```python
from build123d import *

# Parameters (mm, degrees)
CROQUIS1_W                       = 580
CROQUIS1_H                       = 8.5
CROQUIS4_R                       = 9.75
SALIENTE_EXTRUIR1_DEPTH          = 4
MATRIZL1_COUNT                   = 2
MATRIZL1_PITCH                   = 442
SALIENTE_EXTRUIR3_DEPTH          = 3.8
MATRIZL2_COUNT                   = 2
MATRIZL2_PITCH                   = 40
MATRIZL3_COUNT                   = 2
MATRIZL3_PITCH                   = 332
MATRIZL3_COPY_1_DEPTH            = 3.8
CROQUIS6_R                       = 8.5
SALIENTE_EXTRUIR4_DEPTH          = 3.8
MATRIZL4_COUNT                   = 2
MATRIZL4_PITCH                   = 40
MATRIZL5_COUNT                   = 2
MATRIZL5_PITCH                   = 110
MATRIZL5_COPY_1_SKETCH_R         = 8.5
MATRIZL5_COPY_1_DEPTH            = 3.8
CROQUIS7_R                       = 9.75
CORTAR_EXTRUIR1_DEPTH            = 12
CROQUIS8_R                       = 9.75
SALIENTE_EXTRUIR5_DEPTH          = 4
CROQUIS9_R                       = 8.5
SALIENTE_EXTRUIR6_DEPTH          = 8
CHAFL_N1_SIZE                    = 1
SALIENTE_EXTRUIR7_DEPTH          = 5
SALIENTE_EXTRUIR7_DEPTH_BACK     = 5
CROQUIS10_R                      = 15
CROQUIS11_W                      = 6
CROQUIS11_H                      = 3.35
SALIENTE_EXTRUIR8_DEPTH          = 40
CORTAR_EXTRUIR2_START            = -68.25
CROQUIS12_R                      = 42.065931182
CORTAR_EXTRUIR2_DEPTH            = 68.25
TALADRO_DE_MARGEN_PARA_M71_D     = 7.6
TALADRO_DE_MARGEN_PARA_M71_DEPTH = 30
TALADRO_DE_MARGEN_PARA_M71_TIP   = 2.283270352


with BuildPart() as part:
    # Croquis1 → Revolución1 (revolve)
    with BuildSketch(Plane.XY, mode=Mode.PRIVATE) as revoluci_n1_sk:
        with Locations((290, 4.25)):
            Rectangle(CROQUIS1_W, CROQUIS1_H)
    revolve(revoluci_n1_sk.sketch.rotate(Axis((0, 8.5, 0), (1, 0, 0)), 270), axis=Axis((0, 8.5, 0), (1, 0, 0)))

    # Croquis4 → Saliente-Extruir1 (add)
    with BuildSketch(Plane(origin=(580, 0, 0), x_dir=(0, 0, -1), z_dir=(1, 0, 0))):
        with Locations((0, 8.5)):
            Circle(CROQUIS4_R)
    saliente_extruir1 = extrude(amount=-SALIENTE_EXTRUIR1_DEPTH)

    # MatrizL1: Saliente-Extruir1 ×2
    with Locations(*[(-i * MATRIZL1_PITCH, 0, 0) for i in range(1, MATRIZL1_COUNT)]):
        add(saliente_extruir1)

    # Croquis5 → Saliente-Extruir3 (add, symmetric)
    with BuildSketch(Plane(origin=(171, 0, 0), x_dir=(0, 0, -1), z_dir=(1, 0, 0))):
        with BuildLine():
            ThreePointArc((-8.57686354, 11.227161863), (0, -0.5), (8.57686354, 11.227161863))
            ThreePointArc((8.57686354, 11.227161863), (6.71423124, 16.165722115), (4.341375372, 20.880415264))
            ThreePointArc((4.341375372, 20.880415264), (0, 23.4), (-4.341375372, 20.880415264))
            ThreePointArc((-4.341375372, 20.880415264), (-6.71423124, 16.165722115), (-8.57686354, 11.227161863))
        make_face()
    saliente_extruir3 = extrude(amount=SALIENTE_EXTRUIR3_DEPTH, both=True)

    # MatrizL2: Saliente-Extruir3 ×2
    with Locations(*[(i * MATRIZL2_PITCH, 0, 0) for i in range(1, MATRIZL2_COUNT)]):
        add(saliente_extruir3)

    # MatrizL3: Saliente-Extruir3 ×2
    with Locations(*[(i * MATRIZL3_PITCH, 0, 0) for i in range(1, MATRIZL3_COUNT)]):
        add(saliente_extruir3)

    # MatrizL3 copy 1 sketch → MatrizL3 copy 1 (add, symmetric)
    with BuildSketch(Plane(origin=(543, 0, 0), x_dir=(0, 0, -1), z_dir=(1, 0, 0))):
        with BuildLine():
            ThreePointArc((-8.57686354, 11.227161863), (0, -0.5), (8.57686354, 11.227161863))
            ThreePointArc((8.57686354, 11.227161863), (6.71423124, 16.165722115), (4.341375372, 20.880415264))
            ThreePointArc((4.341375372, 20.880415264), (0, 23.4), (-4.341375372, 20.880415264))
            ThreePointArc((-4.341375372, 20.880415264), (-6.71423124, 16.165722115), (-8.57686354, 11.227161863))
        make_face()
    extrude(amount=MATRIZL3_COPY_1_DEPTH, both=True)

    # Croquis6 → Saliente-Extruir4 (add, symmetric)
    with BuildSketch(Plane(origin=(281, 0, 0), x_dir=(0, 0, -1), z_dir=(1, 0, 0))):
        with BuildLine():
            ThreePointArc((-12.722376543, 12.627249768), (-14.9, 8.5), (-12.722376543, 4.372750232))
            ThreePointArc((-12.722376543, 4.372750232), (-8.363270987, 1.70804262), (-3.754994824, -0.497917196))
            ThreePointArc((-3.754994824, -0.497917196), (9.75, 8.5), (-3.754994824, 17.497917196))
            ThreePointArc((-3.754994824, 17.497917196), (-8.363270987, 15.29195738), (-12.722376543, 12.627249768))
        make_face()
        with Locations(Location((0, 8.5, 0), (0, 0, 180))):
            Circle(CROQUIS6_R, mode=Mode.SUBTRACT)
    saliente_extruir4 = extrude(amount=SALIENTE_EXTRUIR4_DEPTH, both=True)

    # MatrizL4: Saliente-Extruir4 ×2
    with Locations(*[(i * MATRIZL4_PITCH, 0, 0) for i in range(1, MATRIZL4_COUNT)]):
        add(saliente_extruir4)

    # MatrizL5: Saliente-Extruir4 ×2
    with Locations(*[(i * MATRIZL5_PITCH, 0, 0) for i in range(1, MATRIZL5_COUNT)]):
        add(saliente_extruir4)

    # MatrizL5 copy 1 sketch → MatrizL5 copy 1 (add, symmetric)
    with BuildSketch(Plane(origin=(431, 0, 0), x_dir=(0, 0, -1), z_dir=(1, 0, 0))):
        with BuildLine():
            ThreePointArc((-12.722376543, 12.627249768), (-14.9, 8.5), (-12.722376543, 4.372750232))
            ThreePointArc((-12.722376543, 4.372750232), (-8.363270987, 1.70804262), (-3.754994824, -0.497917196))
            ThreePointArc((-3.754994824, -0.497917196), (9.75, 8.5), (-3.754994824, 17.497917196))
            ThreePointArc((-3.754994824, 17.497917196), (-8.363270987, 15.29195738), (-12.722376543, 12.627249768))
        make_face()
        with Locations(Location((0, 8.5, 0), (0, 0, 180))):
            Circle(MATRIZL5_COPY_1_SKETCH_R, mode=Mode.SUBTRACT)
    extrude(amount=MATRIZL5_COPY_1_DEPTH, both=True)


with BuildPart() as body_2:
    # Simetría1: mirrored copy
    add(part.part.mirror(Plane.ZY))

    # Croquis7 → Cortar-Extruir1 (cut)
    with BuildSketch(Plane.ZY.offset(580)):
        with Locations(Location((0, 8.5, 0), (0, 0, 180))):
            Circle(CROQUIS7_R)
    extrude(amount=-CORTAR_EXTRUIR1_DEPTH, mode=Mode.SUBTRACT)

    # Croquis8 → Saliente-Extruir5 (add)
    with BuildSketch(Plane.ZY.offset(568)):
        with Locations(Location((0, 8.5, 0), (0, 0, 180))):
            Circle(CROQUIS8_R)
    extrude(amount=SALIENTE_EXTRUIR5_DEPTH)

    # Croquis9 → Saliente-Extruir6 (add)
    with BuildSketch(Plane.ZY.offset(572)):
        with Locations((0, 8.5)):
            Circle(CROQUIS9_R)
    extrude(amount=SALIENTE_EXTRUIR6_DEPTH)

    # Chaflán1
    chafl_n1_edges = [body_2.edges().sort_by_distance(p)[0] for p in [
        (-580, 8.5, -8.5),
    ]]
    chamfer(chafl_n1_edges, length=CHAFL_N1_SIZE)

    # Croquis10 → Saliente-Extruir7 (add, two sides: drawn at the far end of the back side and taken through both)
    with BuildSketch(Plane(origin=(-100.25, 0, 0), x_dir=(0, 0, -1), z_dir=(1, 0, 0)).offset(-SALIENTE_EXTRUIR7_DEPTH_BACK)):
        with Locations((0, 8.5)):
            Circle(CROQUIS10_R)
    extrude(amount=SALIENTE_EXTRUIR7_DEPTH + SALIENTE_EXTRUIR7_DEPTH_BACK)

    # Croquis11 → Saliente-Extruir8 (add)
    with BuildSketch(Plane(origin=(-95.25, 0, 0), x_dir=(0, 0, -1), z_dir=(1, 0, 0))):
        with Locations((0, 18.12798686)):
            Rectangle(CROQUIS11_W, CROQUIS11_H)
    extrude(amount=SALIENTE_EXTRUIR8_DEPTH)

    # Croquis12 → Cortar-Extruir2 (cut)
    with BuildSketch(Plane(origin=(0, 0, 0), x_dir=(0, 0, -1), z_dir=(1, 0, 0)).offset(CORTAR_EXTRUIR2_START)):
        with Locations((0, 8.5)):
            Circle(CROQUIS12_R)
    extrude(amount=CORTAR_EXTRUIR2_DEPTH, mode=Mode.SUBTRACT)

    # Taladro de margen para M71
    with Locations(Plane(origin=(-68.25, 8.5, 0), x_dir=(0, 0, 1), z_dir=(1, 0, 0))):
        with Locations((0, 0)):
            Hole(TALADRO_DE_MARGEN_PARA_M71_D / 2, depth=TALADRO_DE_MARGEN_PARA_M71_DEPTH)
            with Locations((0, 0, -(TALADRO_DE_MARGEN_PARA_M71_DEPTH + TALADRO_DE_MARGEN_PARA_M71_TIP / 2))):  # 118° drill point
                Cone(0, TALADRO_DE_MARGEN_PARA_M71_D / 2, TALADRO_DE_MARGEN_PARA_M71_TIP, mode=Mode.SUBTRACT)


solid = body_2.part
```
Part model, mm, in its own coordinate system. A direction names the side the tool comes from. Give positions to 0.01 mm unless a question says otherwise; leave off trailing zeros. Write each loop counter-clockwise with the first axis right and the second up, starting at its lowest first coordinate (ties: lowest second). Pieces come first, ordered by that corner, then holes. Notation, with made-up numbers: (-26, 73.5) -> (26, 73.5) arc R21 ccw to (26, 96.5) -> close; hole circle Ø10 at (28.25, -9). An arc over 180 degrees is marked (long way). Put each result on its own line as item: value. Start each with the question number.
Item 1: Which spindle directions (+Z, -Z, +X, -X, +Y, -Y) get a long thin tool onto all of the face, cutting with end or side? Do faces 1 (the face through (-580, 9, 0)), 2 (the face through (-434.8, 9, 9)), 3 (the face through (-569.972, -1.167, 1.269)). Say none if no direction does.
Item 2: Pull direction X, two halves, no side cores. Call faces 4 (the face through (-68.25, 12, -2)), 5 (the face through (-575.45, 0.2, -1.84)), 6 (the face through (-394.8, 9, 9)): pulls with the +X half, pulls with the -X half, needs draft (parallel to the pull), parting line crosses it, or undercut.
Item 3: Wall check: L1, parallel to X at y = 6, z = 13.5; L2, parallel to Y at x = -87, z = 0; L3, parallel to Y at x = -373, z = 0.25. Give the ranges that are in metal, low to high. Write a range as [from, to].
Item 4: Pin check, flat tips, straight feed: pin 1 Ø10 at (x, z) = (-174, 1.5) entering from -Y; pin 2 Ø15.5 at (y, z) = (6, -2) entering from +X; pin 3 Ø2.5 at (x, y) = (-75.5, 17.5) entering from +Z; pin 4 Ø4 at (y, z) = (7.5, 11) entering from -X. Stop position of each tip, or through.
Item 5: Cut at A-A (x = -519). List the corners of the cut face in (y, z), then the cut area to 3 significant figures.
Answer list:
1. face 1: +Z, -Z, -X, +Y, -Y
1. face 2: none
1. face 3: -X
2. face 4: pulls with the +X half
2. face 5: needs draft
2. face 6: undercut
3. L1: x = [-434.8, -427.2], [-394.8, -387.2], [-324.8, -317.2], [-284.8, -277.2], [-105.25, -95.25]
3. L2: y = [0, 4.7], [12.3, 19.8]
3. L3: y = [0, 17]
4. pin 1: stops at y = -0.5
4. pin 2: stops at x = -68.25
4. pin 3: stops at z = 3.49
4. pin 4: stops at x = -572
5. outline: circle Ø17 at (8.5, 0)
5. area: 227 mm2
